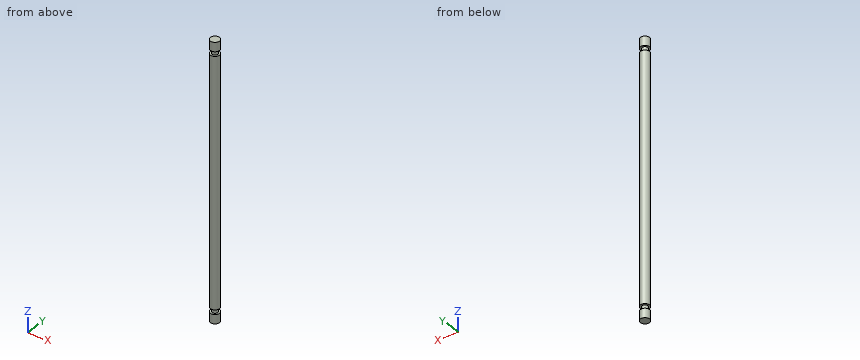
from build123d import *

# Parameters (mm, degrees)
SKETCH2_W = 1.27
SKETCH2_H = 76.2
SKETCH3_W = 0.499412869
SKETCH3_H = 1.27


with BuildPart() as part:
    # Sketch2 → Revolve1 (revolve)
    with BuildSketch(Plane(origin=(0, 0, 0), x_dir=(1, 0, 0), z_dir=(0, 1, 0))):
        with Locations((0.635, 38.1)):
            Rectangle(SKETCH2_W, SKETCH2_H)
    revolve(axis=Axis((0, 0, 0), (0, 0, -1)))

    # Sketch3 → Cut-Revolve1 (revolve, cut)
    with BuildSketch(Plane(origin=(0, 0, 0), x_dir=(1, 0, 0), z_dir=(0, 1, 0))):
        with Locations((1.020293566, 3.175)):
            Rectangle(SKETCH3_W, SKETCH3_H)
    cut_revolve1 = revolve(axis=Axis((0, 0, 0), (0, 0, -1)), mode=Mode.SUBTRACT)

    # Mirror1: Cut-Revolve1 across plane
    add(cut_revolve1.mirror(Plane.XY.offset(-38.1)), mode=Mode.SUBTRACT)


solid = part.part
Design review of the part built by this model. Coordinates are the model's own, in mm. Round coordinates to 2 decimals unless told otherwise and drop trailing zeros. Write each loop counter-clockwise with the first axis right and the second up, starting at its lowest first coordinate (ties: lowest second). Pieces come first, ordered by that corner, then holes.
Item 1: For pin 1 Ø1 at (y, z) = (1, -47.5) entering from -X; pin 2 Ø1 at (y, z) = (-1, -27) entering from +X, all flat-tipped, find the tip position at first contact; note any pin that passes through.
Item 2: Consider section A-A on x = -0.3. Give the boundary of the cut face in (y, z).
Item 3: Consider section B-B on z = -32.5. Give the boundary of the cut face in (x, y), and give its area (3 significant figures).
Item 4: Wall thickness on L1, parallel to Z at x = -0.8, y = -0.5; L2, parallel to X at y = -0.1, z = -27.5; L3, parallel to Y at x = -1, z = -10.5: over which ranges is each line inside the solid? List them lowest first.
Check values:
1. pin 1: stops at x = -1.17
1. pin 2: stops at x = 1.17
2. outline: (-1.23, -76.2) - (1.23, -76.2) - (1.23, -73.66) - (0.71, -73.66) - (0.71, -72.39) - (1.23, -72.39) - (1.23, -3.81) - (0.71, -3.81) - (0.71, -2.54) - (1.23, -2.54) - (1.23, 0) - (-1.23, 0) - (-1.23, -2.54) - (-0.71, -2.54) - (-0.71, -3.81) - (-1.23, -3.81) - (-1.23, -72.39) - (-0.71, -72.39) - (-0.71, -73.66) - (-1.23, -73.66) - close
3. outline: circle Ø2.54 at (0, 0)
3. area: 5.07 mm2
4. L1: z = -76.2 to -73.66, -72.39 to -3.81, -2.54 to 0
4. L2: x = -1.27 to 1.27
4. L3: y = -0.78 to 0.78
